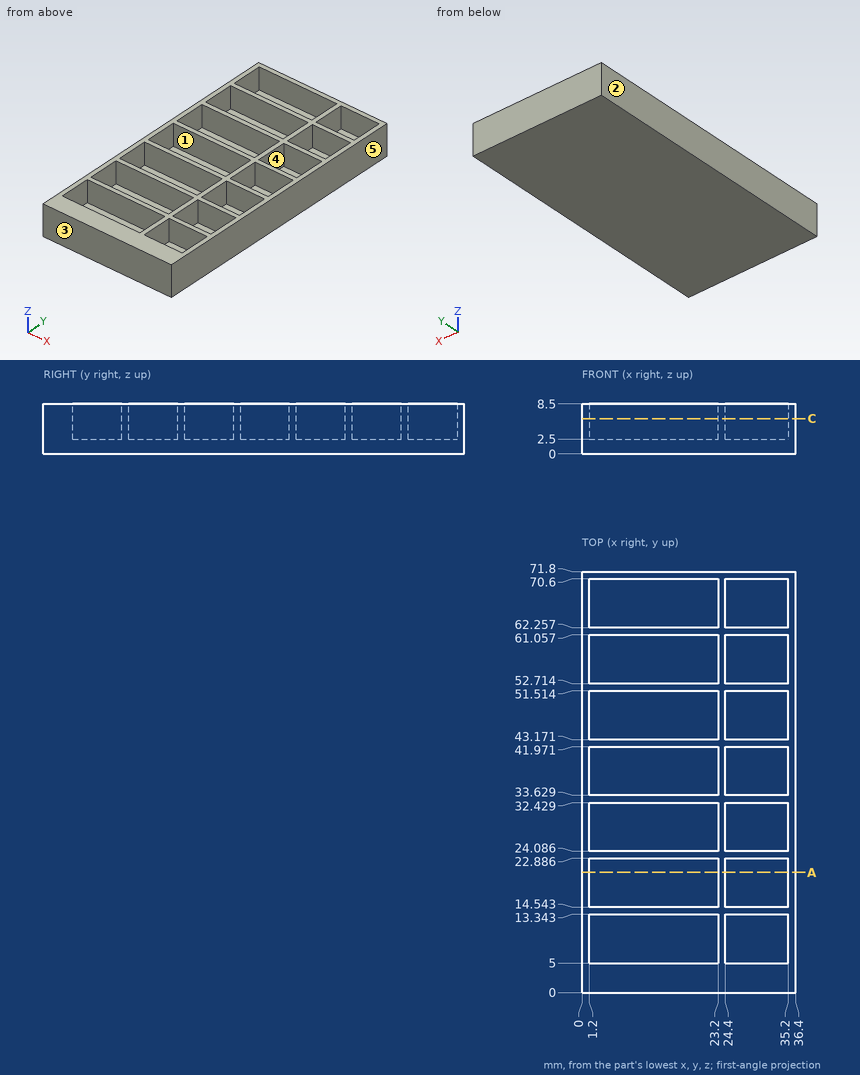
For this review, use the dimensioned drawing (mm, ordinates from the lowest corner) and the shaded views. A direction names the side the tool comes from. Round coordinates to 2 decimals unless told otherwise and drop trailing zeros. Loops run counter-clockwise (first coordinate to the right, second up) from the corner with the lowest first, then second, coordinate; pieces in that order, holes last. Notation, with made-up numbers: M 87.5,-3.75 L 120.5,-3.75 A11 ccw 120.5,1.25 Z; hole C 75,-19.5 d4. An arc over 180 degrees is marked long. Answer as a JSON object with one key per item and string values.
(1) To check wall thickness, follow line 1 along X through (y, z) = (21, 7); line 2 along Z through (x, y) = (13.5, 54.5). State the ranges of each line that lie inside material, in increasing order.
Resolved:
{"line 1": "0 to 1.2, 23.2 to 24.4, 35.2 to 36.4", "line 2": "0 to 2.5"}
(2) Take a section at C-C on z = 6. Count the separate pieces of the cut face and the enclosed holes in it.
Resolved:
{"separate pieces": "1", "enclosed holes": "14"}
(3) Tool access review of the marked faces 1 and 2: name each direction out of +Z, -Z, +X, -X, +Y, -Y from which nothing blocks a thin tool from reaching the whole face with its end or side.
Resolved:
{"face 1": "+Z", "face 2": "+Z, -Z, -X, +Y, -Y"}
(4) Clearance check with a flat-ended pin moving along its axis: P1, Ø4, axis at x = 31, y = 36, coming from the +Z side. State where the tip first meets the part, or that it passes through.
Resolved:
{"P1": "z = 2.5"}
(5) Draft analysis for pull direction Y (two halves, no side actions). For the marked faces 3, 4 and 5, state which applies: released by +Y, released by -Y, zero draft, split by the parting line, or undercut.
Resolved:
{"face 3": "released by -Y", "face 4": "undercut", "face 5": "zero draft"}
(6) Take a section at A-A on y = 20.5. Give the boundary of the cut face in (x, z).
Resolved:
{"outline": "M 0,0 L 36.4,0 L 36.4,8.5 L 35.2,8.5 L 35.2,2.5 L 24.4,2.5 L 24.4,8.5 L 23.2,8.5 L 23.2,2.5 L 1.2,2.5 L 1.2,8.5 L 0,8.5 Z"}
